Geometry check sheet. Reference: the model listing, model coordinates, mm. A direction names the side the tool comes from. Round coordinates to 2 decimals unless told otherwise and drop trailing zeros. Write each loop counter-clockwise with the first axis right and the second up, starting at its lowest first coordinate (ties: lowest second). Pieces come first, ordered by that corner, then holes. Notation, with made-up numbers: (16, 8.25) - (28, 8.25) arc R3 ccw to (28, 13.25) - close; hole circle Ø4 at (-22.5, 66.5). An arc over 180 degrees is marked (long way). Return JSON: item names as keys, results as strings.
```python
from build123d import *

# Parameters (mm, degrees)
SKETCH1_R          = 27.5
SKETCH1_R_2        = 25
SKETCH1_R_3        = 20.5
BASE_EXTRUDE_DEPTH = 10


with BuildPart() as part:
    # Sketch1 → Base-Extrude (new body)
    with BuildSketch(Plane.XY):
        with BuildLine():
            Line((7.049670091, -79.688783098), (345.287252568, -49.766587323))
            ThreePointArc((345.287252568, -49.766587323), (355.557216326, -47.948019985), (365.357095704, -44.378467222))
            Line((365.357095704, -44.378467222), (459.062839102, -0.682761463))
            ThreePointArc((459.062839102, -0.682761463), (475.969488221, 5.056272584), (493.717536564, 7))
            Line((493.717536564, 7), (664.517065511, 7))
            ThreePointArc((664.517065511, 7), (678.75621608, 5.754235747), (692.562717264, 2.054794904))
            Line((692.562717264, 2.054794904), (729.4787914, -11.381557247))
            ThreePointArc((729.4787914, -11.381557247), (757.831571533, -14.486691682), (784.414586181, -4.149122657))
            Line((784.414586181, -4.149122657), (984.431516581, 135.904239779))
            ThreePointArc((984.431516581, 135.904239779), (986.332219153, 141.503528998), (981.5636344, 145))
            Line((981.5636344, 145), (784.07485266, 145))
            ThreePointArc((784.07485266, 145), (732.771831161, 154.046106882), (687.656711207, 180.093333532))
            Line((687.656711207, 180.093333532), (683.783141558, 183.343644395))
            ThreePointArc((683.783141558, 183.343644395), (659.677118187, 191.998591153), (635.725815927, 182.924254468))
            Line((635.725815927, 182.924254468), (596.111500497, 148.488055437))
            ThreePointArc((596.111500497, 148.488055437), (557.515006487, 124.135481312), (513.381915638, 112.516208165))
            Line((513.381915638, 112.516208165), (378.657265123, 98.356076801))
            ThreePointArc((378.657265123, 98.356076801), (337.418162835, 107.87687375), (310.782894659, 140.768690684))
            Line((310.782894659, 140.768690684), (305.217826435, 156.058589967))
            ThreePointArc((305.217826435, 156.058589967), (313.65566679, 220.150350545), (370.99630989, 250))
            Line((370.99630989, 250), (415.871293046, 250))
            ThreePointArc((415.871293046, 250), (442.01801587, 248.858409428), (467.965746346, 245.442325904))
            Line((467.965746346, 245.442325904), (534.131759112, 233.775472647))
            ThreePointArc((534.131759112, 233.775472647), (539.698463104, 236.989410696), (537.5, 243.029638431))
            Line((537.5, 243.029638431), (456.478157281, 289.807621135))
            ThreePointArc((456.478157281, 289.807621135), (384.123870812, 319.777747887), (306.478157281, 330))
            Line((306.478157281, 330), (233.431457505, 330))
            ThreePointArc((233.431457505, 330), (218.12412021, 326.9551813), (205.147186258, 318.284271247))
            Line((205.147186258, 318.284271247), (-56.568542495, 56.568542495))
            ThreePointArc((-56.568542495, 56.568542495), (-72.488236118, -33.844580431), (7.049670091, -79.688783098))
        make_face()
        Circle(SKETCH1_R, mode=Mode.SUBTRACT)
        with Locations((340, 10)):
            Circle(SKETCH1_R_2, mode=Mode.SUBTRACT)
        with Locations((750, 45)):
            Circle(SKETCH1_R_2, mode=Mode.SUBTRACT)
        with Locations((660, 155)):
            Circle(SKETCH1_R_3, mode=Mode.SUBTRACT)
    extrude(amount=-BASE_EXTRUDE_DEPTH)


solid = part.part
```
(1) Release check for a two-part mould opening along X. For faces 1 (the face through (883.023, 64.897, -4.93)), 2 (the face through (616.2, 165.95, -4.93)), 3 (the face through (327, 82, -10)), 4 (the face through (337.93, 107.56, -4.93)) record: pulls with the +X half, pulls with the -X half, needs draft (parallel to the pull), parting line crosses it, or undercut.
Response values:
{"face 1": "pulls with the +X half", "face 2": "undercut", "face 3": "needs draft", "face 4": "undercut"}
(2) Access from +Z, -Z, +X, -X, +Y, -Y to the whole of each face (thin tool, end or side, straight path). Record for faces 5 (the face through (411.55, -22.84, -4.93)), 6 (the face through (733.461, 153.797, -4.93)), 7 (the face through (313.121, 219.376, -4.93)).
Response values:
{"face 5": "+Z, -Z, -Y", "face 6": "+Z, -Z, +X, +Y", "face 7": "+Z, -Z"}
(3) Section check C-C, the plane y = 302. Enter the section's corners in (x, z).
Response values:
{"outline": "(188.86, -10) - (433.03, -10) - (433.03, 0) - (188.86, 0) - close"}
(4) Section check D-D, the plane x = 572. Enter the section's corners in (y, z), plus the area to 3 significant figures.
Response values:
{"outline": "(7, -10) - (131.39, -10) - (131.39, 0) - (7, 0) - close", "area": "1,240 mm^2"}
(5) Section check A-A, the plane z = -6.5. Give the number of separate pieces and of enclosed holes in the cut face, plus the area to 3 significant figures.
Response values:
{"separate pieces": "1", "enclosed holes": "4", "area": "198,000 mm^2"}
(6) Gauge pin test, flat ends, axial feed: pin 1 (1.5 mm diameter, centred on x = 488, z = -6, fed in from +Y); pin 2 (6 mm diameter, centred on y = 19.5, z = -5.5, fed in from -X); pin 3 (5 mm diameter, centred on x = 383.5, z = -5, fed in from -Y). Record the tip position at first contact, or that the pin passes through.
Response values:
{"pin 1": "stops at y = 272.04", "pin 2": "stops at x = -78.28", "pin 3": "stops at y = -37.08"}
(7) Section check B-B, the plane x = 750. Enter the section's corners in (y, z), plus the area to 3 significant figures.
Response values:
{"outline": "(-15, -10) - (20, -10) - (20, 0) - (-15, 0) - close; (70, -10) - (148.92, -10) - (148.92, 0) - (70, 0) - close", "area": "1,140 mm^2"}
(8) Material ranges on line 1 along Y through (x, z) = (340, -5.25); line 2 along Y through (x, z) = (660, -2.75); line 3 along Y through (x, z) = (0, -4.5), recorded low to high. Write a range as [from, to].
Response values:
{"line 1": "y = [-50.23, -15], [35, 106.35], [242.76, 328.12]", "line 2": "y = [7, 134.5], [175.5, 192]", "line 3": "y = [-80, -27.5], [27.5, 113.14]"}
